from build123d import *

# Parameters (mm, degrees)
F0_W     = 697.8
F0_H     = 50.8
F0_R     = 2.5527
F1_DEPTH = 25.4
F2_W     = 47.625
F2_H     = 22.225
F3_DEPTH = 697.801
F4_R     = 2.5527
F5_DEPTH = 25.4


with BuildPart() as f1:
    # F0 (on Top) → F1 (new body)
    with BuildSketch(Plane.XY):
        Rectangle(F0_W, F0_H)
        with Locations((-336.2, -12.7)):
            Circle(F0_R, mode=Mode.SUBTRACT)
        with Locations((-336.2, 0)):
            Circle(F0_R, mode=Mode.SUBTRACT)
        with Locations((336.2, -12.7)):
            Circle(F0_R, mode=Mode.SUBTRACT)
        with Locations((336.2, 0)):
            Circle(F0_R, mode=Mode.SUBTRACT)
        with Locations((-336.2, 12.7)):
            Circle(F0_R, mode=Mode.SUBTRACT)
        with Locations((336.2, 12.7)):
            Circle(F0_R, mode=Mode.SUBTRACT)
    extrude(amount=F1_DEPTH)

    # F2 (on face) → F3 (cut, through all)
    with BuildSketch(Plane(origin=(-348.9, 0, 0), x_dir=(0, -1, 0), z_dir=(-1, 0, 0))):
        with Locations((0, 12.7)):
            Rectangle(F2_W, F2_H)
    extrude(amount=-F3_DEPTH, mode=Mode.SUBTRACT)

    # F4 (on face) → F5 (cut)
    with BuildSketch(Plane.XY.offset(25.4)):
        with Locations((-227.8436, 12.7)):
            Circle(F4_R)
        with Locations((-227.8436, -12.7)):
            Circle(F4_R)
        with Locations((-260, -12.7)):
            Circle(F4_R)
        with Locations((-260, 12.7)):
            Circle(F4_R)
        with Locations((227.8436, 12.7)):
            Circle(F4_R)
        with Locations((260, -12.7)):
            Circle(F4_R)
        with Locations((227.8436, -12.7)):
            Circle(F4_R)
        with Locations((260, 12.7)):
            Circle(F4_R)
    extrude(amount=-F5_DEPTH, mode=Mode.SUBTRACT)


solid = f1.part
Check sheet for the modelled part. Datum: model origin and axes. Units: mm. A direction names the side the tool comes from. Round coordinates to 2 decimals unless told otherwise and drop trailing zeros. Write each loop counter-clockwise with the first axis right and the second up, starting at its lowest first coordinate (ties: lowest second). Pieces come first, ordered by that corner, then holes. Notation, with made-up numbers: (65.25, -4) -> (124.25, -4) arc R19 ccw to (124.25, 19) -> close; hole circle Ø9 at (15, 83). An arc over 180 degrees is marked (long way). Answer as CSV lines item,"result". Start each with the question number.
1) Tool access check on faces 4 (the flat face through (-348.9, -2, 24)), 5 (the flat face through (-5, -23.812, 13)). Record the directions out of +Z, -Z, +X, -X, +Y, -Y that give a thin tool (end or side, any length) a straight path to the whole face; none if there is none.
2) Section check B-B on x = 51. Enter the section's corners in (y, z), and give its area (3 significant figures).
3) Section check A-A on z = 7.25. Enter the section's corners in (x, y), and give its area (3 significant figures).
4) Release check for a two-part mould opening along Z. For faces 1 (the flat face through (-5, 0, 25.4)), 2 (the flat face through (-5, -25.4, 13)), 3 (the flat face through (-5, 0, 23.812)) record: pulls with the +Z half, pulls with the -Z half, needs draft (parallel to the pull), parting line crosses it, or undercut.
5) Go/stop test with a flat-tipped pin: P1, Ø3, axis at x = -227.84, y = 12.7, coming from the +Z side. Record where the tip stops, or that it passes through.
6) Material ranges on line 1 (Y direction, x = 336.2, z = 24.6); line 2 (X direction, y = 0, z = 1.2); line 3 (Z direction, x = 189, y = 6), recorded low to high. Write a range as from..to.
Found:
1,face 4,"+Z, -Z, -X, +Y, -Y"
1,face 5,"+X, -X"
2,outline,"(-25.4, 0) -> (25.4, 0) -> (25.4, 25.4) -> (-25.4, 25.4) -> close; hole (-23.81, 1.59) -> (23.81, 1.59) -> (23.81, 23.81) -> (-23.81, 23.81) -> close"
2,area,"232 mm^2"
3,outline,"(-348.9, -25.4) -> (348.9, -25.4) -> (348.9, -23.81) -> (-348.9, -23.81) -> close; (-348.9, 23.81) -> (348.9, 23.81) -> (348.9, 25.4) -> (-348.9, 25.4) -> close"
3,area,"2,220 mm^2"
4,face 1,"pulls with the +Z half"
4,face 2,"needs draft"
4,face 3,"undercut"
5,P1,"passes through"
6,line 1,"y = -25.4..-15.25, -10.15..-2.55, 2.55..10.15, 15.25..25.4"
6,line 2,"x = -348.9..-338.75, -333.65..333.65, 338.75..348.9"
6,line 3,"z = 0..1.59, 23.81..25.4"
